Verification items for the finished model (mm, model axes). Coordinates: 2 decimals unless noted, no trailing zeros. Write each loop counter-clockwise with the first axis right and the second up, starting at its lowest first coordinate (ties: lowest second). Pieces come first, ordered by that corner, then holes. Notation, with made-up numbers: (-5, 54.5) -> (26, 54.5) arc R25 ccw to (26, 84.5) -> close; hole circle Ø11 at (-8, 13.5). An arc over 180 degrees is marked (long way). Answer in a Markdown table with one row per item.
```python
from build123d import *

# Parameters (mm, degrees)
EXTRUDE_THIN1_DEPTH = 50
SKETCH3_R           = 14
CUT_EXTRUDE2_DEPTH  = 10
CUT_EXTRUDE3_REACH  = 135.651
SKETCH4_W           = 129.958556301
SKETCH4_H           = 19.187259519


with BuildPart() as part:
    # Sketch1 → Extrude-Thin1 (new, symmetric)
    with BuildSketch(Plane(origin=(0, 0, 0), x_dir=(1, 0, 0), z_dir=(0, 1, 0))):
        with BuildLine():
            Line((-57.5, 60), (-57.5, -60))
            ThreePointArc((-57.5, -60), (-55.303300859, -65.303300859), (-50, -67.5))
            Line((-50, -67.5), (50, -67.5))
            ThreePointArc((50, -67.5), (55.303300859, -65.303300859), (57.5, -60))
            Line((57.5, -60), (57.5, 60))
            ThreePointArc((57.5, 60), (55.303300859, 65.303300859), (50, 67.5))
            Line((50, 67.5), (-50, 67.5))
            ThreePointArc((-50, 67.5), (-55.303300859, 65.303300859), (-57.5, 60))
        make_face()
        with BuildLine():
            Line((-52.5, 60), (-52.5, -60))
            ThreePointArc((-52.5, -60), (-51.767766953, -61.767766953), (-50, -62.5))
            Line((-50, -62.5), (50, -62.5))
            ThreePointArc((50, -62.5), (51.767766953, -61.767766953), (52.5, -60))
            Line((52.5, -60), (52.5, 60))
            ThreePointArc((52.5, 60), (51.767766953, 61.767766953), (50, 62.5))
            Line((50, 62.5), (-50, 62.5))
            ThreePointArc((-50, 62.5), (-51.767766953, 61.767766953), (-52.5, 60))
        make_face(mode=Mode.SUBTRACT)
    extrude(amount=EXTRUDE_THIN1_DEPTH, both=True)

    # Sketch3 → Cut-Extrude2 (cut)
    with BuildSketch(Plane(origin=(0, 0, -67.5), x_dir=(-1, 0, 0), z_dir=(0, 0, -1))):
        Circle(SKETCH3_R)
    extrude(amount=-CUT_EXTRUDE2_DEPTH, mode=Mode.SUBTRACT)

    # Sketch4 → Cut-Extrude3 (cut, up to next)
    with BuildSketch(Plane(origin=(0, 50, 0), x_dir=(1, 0, 0), z_dir=(0, 1, 0)), mode=Mode.PRIVATE) as cut_extrude3_sk1:
        with Locations((-6.555772869, -70.09362976)):
            Rectangle(SKETCH4_W, SKETCH4_H)
    cut_extrude3_tool1 = extrude(cut_extrude3_sk1.sketch, amount=-CUT_EXTRUDE3_REACH, mode=Mode.PRIVATE) & part.part
    add(cut_extrude3_tool1.solids().sort_by_distance((-6.555773, 50, 70.09363))[0], mode=Mode.SUBTRACT)


solid = part.part
```
1. Section check C-C, the plane z = 29. Record the boundary of the cut face in (x, y).
Geometry says:
| item | result |
|---|---|
| outline | (-57.5, -50) -> (-52.5, -50) -> (-52.5, 50) -> (-57.5, 50) -> close; (52.5, -50) -> (57.5, -50) -> (57.5, 50) -> (52.5, 50) -> close |
2. Section check D-D, the plane y = 22.5. Record the boundary of the cut face in (x, z).
Geometry says:
| item | result |
|---|---|
| outline | (-57.5, -60) arc R7.5 ccw to (-50, -67.5) -> (50, -67.5) arc R7.5 ccw to (57.5, -60) -> (57.5, 60) arc R7.5 ccw to (57.48, 60.5) -> (52.45, 60.5) arc R2.5 cw to (52.5, 60) -> (52.5, -60) arc R2.5 cw to (50, -62.5) -> (-50, -62.5) arc R2.5 cw to (-52.5, -60) -> (-52.5, 60) arc R2.5 cw to (-52.45, 60.5) -> (-57.48, 60.5) arc R7.5 ccw to (-57.5, 60) -> close |
3. Depth check by flat-ended pin: P1, Ø1.5, axis at x = 8, y = -17, coming from the +Z side. Enter the tip coordinate at first touch or a pass-through.
Geometry says:
| item | result |
|---|---|
| P1 | z = -62.5 |
4. Mould release check, pull along X, two halves, no side actions. Record for faces 1 (the flat face through (57.5, 1, 1)), 2 (the flat face through (0, 50, -65)), 3 (the flat face through (12, 12, -62.5)): released by +X, released by -X, zero draft, split by the parting line, or undercut.
Geometry says:
| item | result |
|---|---|
| face 1 | released by +X |
| face 2 | zero draft |
| face 3 | undercut |
5. Section check B-B, the plane y = 0. Record the boundary of the cut face in (x, z), plus the area to 3 significant figures.
Geometry says:
| item | result |
|---|---|
| outline | (-57.5, -60) arc R7.5 ccw to (-50, -67.5) -> (-14, -67.5) -> (-14, -62.5) -> (-50, -62.5) arc R2.5 cw to (-52.5, -60) -> (-52.5, 60) arc R2.5 cw to (-52.45, 60.5) -> (-57.48, 60.5) arc R7.5 ccw to (-57.5, 60) -> close; (14, -67.5) -> (50, -67.5) arc R7.5 ccw to (57.5, -60) -> (57.5, 60) arc R7.5 ccw to (57.48, 60.5) -> (52.45, 60.5) arc R2.5 cw to (52.5, 60) -> (52.5, -60) arc R2.5 cw to (50, -62.5) -> (14, -62.5) -> close |
| area | 1,640 mm^2 |
6. Section check A-A, the plane x = 0. Record the boundary of the cut face in (y, z).
Geometry says:
| item | result |
|---|---|
| outline | (-50, -67.5) -> (-14, -67.5) -> (-14, -62.5) -> (-50, -62.5) -> close; (14, -67.5) -> (50, -67.5) -> (50, -62.5) -> (14, -62.5) -> close |
7. Thickness scan on line 1 (Y direction, x = 0, z = -64.15); line 2 (X direction, y = -22.5, z = -21); line 3 (Z direction, x = 15, y = 28). Record the ranges inside material, lowest first. Write a range as from..to.
Geometry says:
| item | result |
|---|---|
| line 1 | -50..-14, 14..50 |
| line 2 | -57.5..-52.5, 52.5..57.5 |
| line 3 | -67.5..-62.5 |
